```python
from build123d import *

# Parameters (mm, degrees)
SKETCH1_W               = 20
SKETCH1_H               = 40
BOSS_EXTRUDE1_DEPTH     = 12
CUT_EXTRUDE1_DEPTH      = 43.941821107
CUT_EXTRUDE1_DEPTH_BACK = 43.941821107
CUT_EXTRUDE2_DEPTH      = 43.941821107
CUT_EXTRUDE2_DEPTH_BACK = 43.941821107
SKETCH4_R               = 3
SKETCH4_R_2             = 1.5
BOSS_EXTRUDE2_DEPTH     = 2.5
FILLET1_R               = 1
SKETCH5_R               = 2
BOSS_EXTRUDE3_DEPTH     = 5
BOSS_EXTRUDE4_START     = -5
SKETCH7_R               = 2
BOSS_EXTRUDE4_DEPTH     = 5
FILLET2_R               = 10
SKETCH8_W               = 7
SKETCH8_H               = 6
CUT_EXTRUDE3_DEPTH      = 8
SKETCH10_R              = 2
BOSS_EXTRUDE5_DEPTH     = 7
SKETCH11_W              = 7
SKETCH11_H              = 6
CUT_EXTRUDE4_DEPTH      = 8
SKETCH12_R              = 2
BOSS_EXTRUDE6_DEPTH     = 8
SKETCH13_W              = 4
SKETCH13_H              = 8
CUT_EXTRUDE5_DEPTH      = 6
SKETCH16_W              = 4
SKETCH16_H              = 3
CUT_EXTRUDE6_DEPTH      = 6
SKETCH17_W              = 4
SKETCH17_H              = 8.017766953
CUT_EXTRUDE7_DEPTH      = 52.429563482


with BuildPart() as part:
    # Sketch1 → Boss-Extrude1 (new body)
    with BuildSketch(Plane.XY):
        with Locations((0, -20)):
            Rectangle(SKETCH1_W, SKETCH1_H)
    extrude(amount=BOSS_EXTRUDE1_DEPTH)

    # Sketch2 → Cut-Extrude1 (cut, two sides: drawn at the far end of the back side and taken through both)
    with BuildSketch(Plane(origin=(0, 0, 0), x_dir=(0, 0, -1), z_dir=(1, 0, 0)).offset(-CUT_EXTRUDE1_DEPTH_BACK)):
        Polygon((-8, 0), (0, 0), (0, -8), align=None)
    extrude(amount=CUT_EXTRUDE1_DEPTH + CUT_EXTRUDE1_DEPTH_BACK, mode=Mode.SUBTRACT)

    # Sketch3 → Cut-Extrude2 (cut, two sides: drawn at the far end of the back side and taken through both)
    with BuildSketch(Plane(origin=(0, 0, 0), x_dir=(0, 0, -1), z_dir=(1, 0, 0)).offset(-CUT_EXTRUDE2_DEPTH_BACK)):
        with BuildLine():
            ThreePointArc((-3, 1.1), (-6.559834153, 4.04730143), (-8.791057147, 0))
            Line((-8.791057147, 0), (-7.019803903, 0))
            ThreePointArc((-7.019803903, 0), (-6.600122548, 2.474719218), (-4.5, 1.1))
            ThreePointArc((-4.5, 1.1), (-4.625280782, 0.499877452), (-4.980196097, 0))
            Line((-4.980196097, 0), (-3.208942853, 0))
            ThreePointArc((-3.208942853, 0), (-3.05269857, 0.540165847), (-3, 1.1))
        make_face()
        with BuildLine():
            Line((-7.019803903, 0), (-8.791057147, 0))
            ThreePointArc((-8.791057147, 0), (-6, -1.9), (-3.208942853, 0))
            Line((-3.208942853, 0), (-4.980196097, 0))
            ThreePointArc((-4.980196097, 0), (-6, -0.4), (-7.019803903, 0))
        make_face()
    extrude(amount=CUT_EXTRUDE2_DEPTH + CUT_EXTRUDE2_DEPTH_BACK, mode=Mode.SUBTRACT)

    # Sketch4 → Boss-Extrude2 (add, symmetric)
    with BuildSketch(Plane(origin=(0, 0, 0), x_dir=(0, 0, -1), z_dir=(1, 0, 0))):
        with Locations((-6, 1.1)):
            Circle(SKETCH4_R)
        with Locations((-6, 1.1)):
            Circle(SKETCH4_R_2, mode=Mode.SUBTRACT)
    extrude(amount=BOSS_EXTRUDE2_DEPTH, both=True)

    # Fillet1
    fillet1_edges = [part.edges().sort_by_distance(p)[0] for p in [
        (0, -1.898274836, 6.101725164),
        (0, 0, 8.791057147),
    ]]
    fillet(fillet1_edges, radius=FILLET1_R)

    # Sketch5 → Boss-Extrude3 (add)
    with BuildSketch(Plane(origin=(10, 0, 0), x_dir=(0, 0, -1), z_dir=(1, 0, 0))):
        with BuildLine():
            Line((-2.226818383, -46.327817941), (0, -40))
            Line((0, -40), (-12, -40))
            Line((-12, -40), (-9.773181617, -46.327817941))
            ThreePointArc((-9.773181617, -46.327817941), (-6, -49), (-2.226818383, -46.327817941))
        make_face()
        with Locations(Location((-6, -45, 0), (0, 0, 90))):
            Circle(SKETCH5_R, mode=Mode.SUBTRACT)
    extrude(amount=-BOSS_EXTRUDE3_DEPTH)

    # Sketch7 → Boss-Extrude4 (add)
    with BuildSketch(Plane.ZY.offset(10).offset(BOSS_EXTRUDE4_START)):
        with BuildLine():
            Line((12, -40), (0, -40))
            Line((0, -40), (2.226818383, -46.327817941))
            ThreePointArc((2.226818383, -46.327817941), (6, -49), (9.773181617, -46.327817941))
            Line((9.773181617, -46.327817941), (12, -40))
        make_face()
        with Locations(Location((6, -45, 0), (0, 0, 90))):
            Circle(SKETCH7_R, mode=Mode.SUBTRACT)
    extrude(amount=BOSS_EXTRUDE4_DEPTH)

    # Fillet2
    fillet2_edges = [part.edges().sort_by_distance(p)[0] for p in [
        (0, -8, 0),
    ]]
    fillet(fillet2_edges, radius=FILLET2_R)

    # Sketch8 → Cut-Extrude3 (cut)
    with BuildSketch(Plane.ZY.offset(10)):
        with Locations((6, -29)):
            Rectangle(SKETCH8_W, SKETCH8_H)
    extrude(amount=-CUT_EXTRUDE3_DEPTH, mode=Mode.SUBTRACT)

    # Sketch10 → Boss-Extrude5 (add)
    with BuildSketch(Plane(origin=(0, 0, 9.5), x_dir=(-1, 0, 0), z_dir=(0, 0, -1))):
        with Locations(Location((6, -29, 0), (0, 0, 180))):
            Circle(SKETCH10_R)
    extrude(amount=BOSS_EXTRUDE5_DEPTH)

    # Sketch11 → Cut-Extrude4 (cut)
    with BuildSketch(Plane(origin=(10, 0, 0), x_dir=(0, 0, -1), z_dir=(1, 0, 0))):
        with Locations((-6, -29)):
            Rectangle(SKETCH11_W, SKETCH11_H)
    extrude(amount=-CUT_EXTRUDE4_DEPTH, mode=Mode.SUBTRACT)

    # Sketch12 → Boss-Extrude6 (add)
    with BuildSketch(Plane(origin=(0, 0, 9.5), x_dir=(-1, 0, 0), z_dir=(0, 0, -1))):
        with Locations(Location((-6, -29, 0), (0, 0, 180))):
            Circle(SKETCH12_R)
    extrude(amount=BOSS_EXTRUDE6_DEPTH)

    # Sketch13 → Cut-Extrude5 (cut)
    with BuildSketch(Plane(origin=(0, 0, 0), x_dir=(-1, 0, 0), z_dir=(0, 0, -1))):
        with Locations((0, -33.017766953)):
            Rectangle(SKETCH13_W, SKETCH13_H)
        with Locations((0, -19.088834765)):
            Rectangle(SKETCH13_W, SKETCH13_H)
    extrude(amount=-CUT_EXTRUDE5_DEPTH, mode=Mode.SUBTRACT)

    # Sketch16 → Cut-Extrude6 (cut)
    with BuildSketch(Plane.XZ.offset(29.017766953)):
        with Locations((0, 4.5)):
            Rectangle(SKETCH16_W, SKETCH16_H)
    extrude(amount=-CUT_EXTRUDE6_DEPTH, mode=Mode.SUBTRACT)

    # Sketch17 → Cut-Extrude7 (cut, through all)
    with BuildSketch(Plane(origin=(0, 0, 0), x_dir=(-1, 0, 0), z_dir=(0, 0, -1))):
        with Locations((0, -33.008883477)):
            Rectangle(SKETCH17_W, SKETCH17_H)
    extrude(amount=-CUT_EXTRUDE7_DEPTH, mode=Mode.SUBTRACT)


solid = part.part
```
Part model, mm, in its own coordinate system. A direction names the side the tool comes from. Give positions to 0.01 mm unless a question says otherwise; leave off trailing zeros. Loops run counter-clockwise (first coordinate to the right, second up) from the corner with the lowest first, then second, coordinate; pieces in that order, holes last. Notation, with made-up numbers: M -23,85 L -1,85 A14 ccw -1,104 Z; hole C 79.25,73.5 d2. An arc over 180 degrees is marked long. Return JSON: item names as keys, results as strings.
1) Saw through at D-D, the plane z = 1.25. List the corners of the cut face in (x, y).
Calculated:
{"outline": "M -10,-43.55 L -5,-43.55 L -5,-40 L 5,-40 L 5,-43.55 L 10,-43.55 L 10,-7.3 L -10,-7.3 Z; hole M -2,-37.02 L 2,-37.02 L 2,-29 L -2,-29 Z; hole M -2,-23.09 L 2,-23.09 L 2,-15.09 L -2,-15.09 Z"}
2) 3-axis set-ups, long thin cutter, end or side, ignore diameter. For faces 5 (the face through (2.5, -0.3, 5)), 6 (the face through (-0.1, 0, 10.4)), 7 (the face through (6, -32, 6)), 8 (the face through (-6, -26, 6)), 9 (the face through (-2, -34, 6)): which of +Z, -Z, +X, -X, +Y, -Y reach the whole face in a straight line?
Calculated:
{"face 5": "-Z, +X, +Y", "face 6": "+Z, +Y", "face 7": "+X, -X", "face 8": "-X", "face 9": "+Z, -Z"}
3) Saw through at C-C, the plane x = 0.75. List the corners of the cut face in (y, z) (3 decimals).
Calculated:
{"outline": "M -40,0 L -37.018,0 L -37.018,12 L -40,12 Z; M -29,0 L -23.089,0 L -23.089,3 L -29,3 Z; M -29,6 L -15.089,6 L -15.089,0 L -12.142,0 A10 ccw -5.071,2.929 L -3.15,4.85 A1 cw -1.557,4.607 A3 ccw long 1.025,8.999 A1 cw 0,9.999 L 0,12 L -29,12 Z; hole C 1.1,6 d3"}
4) Pull direction Z, two halves, no side cores. Call faces 1 (the face through (0, -20, 12)), 2 (the face through (7.54, -43.21, 1.13)), 3 (the face through (-7, -47, 6)), 4 (the face through (6, -26, 6)): released by +Z, released by -Z, zero draft, split by the parting line, or undercut.
Calculated:
{"face 1": "released by +Z", "face 2": "released by -Z", "face 3": "undercut", "face 4": "undercut"}
5) Drill centre lines: line 1 (Y direction, x = -6, z = 6); line 2 (X direction, y = -33, z = 10.25); line 3 (Y direction, x = 0.5, z = 10.5). Where is each one in solid material? Low to high.
Calculated:
{"line 1": "y = -49 to -47, -43 to -32, -31 to -27, -26 to -2", "line 2": "x = -10 to -2, 2 to 10", "line 3": "y = -40 to -37.02, -29 to 0"}
6) Saw through at A-A, the plane x = 6. List the corners of the cut face in (y, z).
Calculated:
{"outline": "M -46.33,2.23 L -40,0 L -12.14,0 A10 ccw -5.07,2.93 L -1.9,6.1 A3 cw 0,8.79 L 0,12 L -40,12 L -46.33,9.77 A4 ccw Z; hole C -45,6 d4; hole M -32,2.5 L -31,2.5 L -31,9.5 L -32,9.5 Z; hole M -27,2.5 L -26,2.5 L -26,9.5 L -27,9.5 Z"}
7) Saw through at B-B, the plane y = -45. List the corners of the cut face in (x, z).
Calculated:
{"outline": "M -10,1.76 L -5,1.76 L -5,4 L -10,4 Z; M -10,8 L -5,8 L -5,10.24 L -10,10.24 Z; M 5,1.76 L 10,1.76 L 10,4 L 5,4 Z; M 5,8 L 10,8 L 10,10.24 L 5,10.24 Z"}
8) Flat gauge pins, fed straight in: pin 1 Ø0.9 at (x, z) = (-1, 2) entering from -Y; pin 2 Ø1.5 at (x, y) = (5, -42) entering from -Z; pin 3 Ø3 at (x, z) = (4, 9.5) entering from -Y. Where does each tip first touch, or does it go through?
Calculated:
{"pin 1": "stops at y = -40", "pin 2": "stops at z = 0.44", "pin 3": "stops at y = -48.21"}
